Read the model definition and answer for the solid it produces. Units are mm, in the model's axes. Face numbers are marked on the shaded views. A direction names the side the tool comes from. Give positions to 0.01 mm unless a question says otherwise; leave off trailing zeros. Order: outer loops, then holes, each group sorted by start corner. A loop starts at its lowest first (then second) coordinate and runs counter-clockwise, first axis right, second up. Notation, with made-up numbers: (18.25, -28) - (71.25, -28) arc R19 cw to (71.25, -14) - close; hole circle Ø8 at (-4.75, 7.25). An arc over 180 degrees is marked (long way). One line per item, written item: value. Start each with the question number.
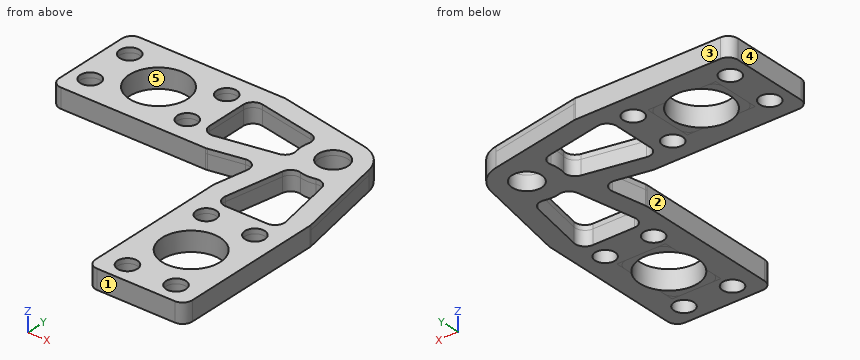
```python
from build123d import *

# Parameters (mm, degrees)
EXTRUDE_1_DEPTH         = 3
SKETCH_2_R              = 2.05
CUT_EXTRUDE_1_DEPTH     = 10
CUT_EXTRUDE_2_DEPTH     = 10
SKETCH_4_R              = 3.05
CUT_EXTRUDE_3_DEPTH     = 10
SKETCH_5_W              = 14
SKETCH_5_H              = 10
SKETCH_5_W_2            = 10
SKETCH_5_H_2            = 14
CUT_EXTRUDE_4_DEPTH     = 10
FILLET_1_R              = 2
FILLET_2_R              = 2
MOVE_START              = 3
MOVE_FACE_1_OUTLINE_R   = 2.05
MOVE_FACE_1_OUTLINE_R_2 = 3.05
MOVE_FACE_1_DEPTH       = 1
SKETCH_9_W              = 14
SKETCH_9_H              = 10
SKETCH_9_W_2            = 10
SKETCH_9_H_2            = 14
EXTRUDE_2_DEPTH         = 4
SKETCH_14_R             = 6
SKETCH_14_R_2           = 2.05
CUT_EXTRUDE_8_DEPTH     = 10


# Read off the part's stored shape, not the designer's step: 移动面1
with BuildPart() as part:
    # 草图1 → 凸台-拉伸1 (new body)
    with BuildSketch(Plane.XY):
        Polygon((-50, 10), (10, 10), (10, -50), (-10, -50), (-10, -10), (-50, -10), align=None)
    extrude(amount=EXTRUDE_1_DEPTH)

    # 草图2 → 切除-拉伸1 (cut)
    with BuildSketch(Plane.XY.offset(3)):
        with Locations((-26, -5)):
            Circle(SKETCH_2_R)
        with Locations((-46, 5)):
            Circle(SKETCH_2_R)
        with Locations((-46, -5)):
            Circle(SKETCH_2_R)
        with Locations((-26, 5)):
            Circle(SKETCH_2_R)
        with Locations((5, -26)):
            Circle(SKETCH_2_R)
        with Locations((-5, -46)):
            Circle(SKETCH_2_R)
        with Locations((5, -46)):
            Circle(SKETCH_2_R)
        with Locations((-5, -26)):
            Circle(SKETCH_2_R)
    extrude(amount=-CUT_EXTRUDE_1_DEPTH, mode=Mode.SUBTRACT)

    # 草图3 → 切除-拉伸2 (cut)
    with BuildSketch(Plane.XY.offset(3)):
        with BuildLine():
            Line((-18, 10), (1.20164514, 6.387961252))
            ThreePointArc((1.20164514, 6.387961252), (4.596194078, 4.596194078), (6.387961252, 1.20164514))
            Line((6.387961252, 1.20164514), (10, -18))
            Line((10, -18), (10, 10))
            Line((10, 10), (-18, 10))
        make_face()
        Polygon((-18, -10), (-8.146437488, -8.146437488), (-10, -18), align=None)
    extrude(amount=-CUT_EXTRUDE_2_DEPTH, mode=Mode.SUBTRACT)

    # 草图4 → 切除-拉伸3 (cut)
    with BuildSketch(Plane.XY.offset(3)):
        Circle(SKETCH_4_R)
    extrude(amount=-CUT_EXTRUDE_3_DEPTH, mode=Mode.SUBTRACT)

    # 草图5 → 切除-拉伸4 (cut)
    with BuildSketch(Plane.XY.offset(3)):
        with Locations((-36, 0)):
            Rectangle(SKETCH_5_W, SKETCH_5_H)
        with BuildLine():
            Line((-22, 6.682287415), (-22, -6.682287415))
            Line((-22, -6.682287415), (-5.43440841, -3.566119072))
            ThreePointArc((-5.43440841, -3.566119072), (-6.5, 0), (-5.43440841, 3.566119072))
            Line((-5.43440841, 3.566119072), (-22, 6.682287415))
        make_face()
        with BuildLine():
            Line((3.566119072, -5.43440841), (6.682287415, -22))
            Line((6.682287415, -22), (-6.682287415, -22))
            Line((-6.682287415, -22), (-3.566119072, -5.43440841))
            ThreePointArc((-3.566119072, -5.43440841), (0, -6.5), (3.566119072, -5.43440841))
        make_face()
        with Locations((0, -36)):
            Rectangle(SKETCH_5_W_2, SKETCH_5_H_2)
    extrude(amount=-CUT_EXTRUDE_4_DEPTH, mode=Mode.SUBTRACT)

    # 圆角1
    fillet_1_edges = [part.edges().sort_by_distance(p)[0] for p in [
        (-29, 5, 1.5),
        (-29, -5, 1.5),
        (-43, -5, 1.5),
        (-43, 5, 1.5),
        (-3.566119072, -5.43440841, 1.5),
        (3.566119072, -5.43440841, 1.5),
        (6.682287415, -22, 1.5),
        (-6.682287415, -22, 1.5),
        (5, -43, 1.5),
        (-5, -43, 1.5),
        (-5, -29, 1.5),
        (5, -29, 1.5),
        (-22, 6.682287415, 1.5),
        (-5.43440841, 3.566119072, 1.5),
        (-5.43440841, -3.566119072, 1.5),
        (-22, -6.682287415, 1.5),
    ]]
    fillet(fillet_1_edges, radius=FILLET_1_R)

    # 圆角2
    fillet_2_edges = [part.edges().sort_by_distance(p)[0] for p in [
        (-50, 10, 1.5),
        (10, -50, 1.5),
        (-10, -50, 1.5),
        (-50, -10, 1.5),
        (-18, -10, 1.5),
        (-8.146437488, -8.146437488, 1.5),
        (-10, -18, 1.5),
        (-18, 10, 1.5),
        (10, -18, 1.5),
    ]]
    fillet(fillet_2_edges, radius=FILLET_2_R)

    # Move Face 1 outline → Move Face 1 (add)
    with BuildSketch(Plane.XY.offset(MOVE_START)):
        with BuildLine():
            Line((-50, 8), (-50, -8))
            ThreePointArc((-50, -8), (-49.414213562, -9.414213562), (-48, -10))
            Line((-48, -10), (-18.186475598, -10))
            ThreePointArc((-18.186475598, -10), (-18.000805296, -9.991362985), (-17.816738632, -9.965526539))
            Line((-17.816738632, -9.965526539), (-11.022770604, -8.687507099))
            ThreePointArc((-11.022770604, -8.687507099), (-9.238820076, -9.238820076), (-8.687507099, -11.022770604))
            Line((-8.687507099, -11.022770604), (-9.965526539, -17.816738632))
            ThreePointArc((-9.965526539, -17.816738632), (-9.991362985, -18.000805296), (-10, -18.186475598))
            Line((-10, -18.186475598), (-10, -48))
            ThreePointArc((-10, -48), (-9.414213562, -49.414213562), (-8, -50))
            Line((-8, -50), (8, -50))
            ThreePointArc((8, -50), (9.414213562, -49.414213562), (10, -48))
            Line((10, -48), (10, -18.186475598))
            ThreePointArc((10, -18.186475598), (9.991362985, -18.000805296), (9.965526539, -17.816738632))
            Line((9.965526539, -17.816738632), (6.387961252, 1.20164514))
            ThreePointArc((6.387961252, 1.20164514), (4.596194078, 4.596194078), (1.20164514, 6.387961252))
            Line((1.20164514, 6.387961252), (-17.816738632, 9.965526539))
            ThreePointArc((-17.816738632, 9.965526539), (-18.000805296, 9.991362985), (-18.186475598, 10))
            Line((-18.186475598, 10), (-48, 10))
            ThreePointArc((-48, 10), (-49.414213562, 9.414213562), (-50, 8))
        make_face()
        with Locations((-5, -46)):
            Circle(MOVE_FACE_1_OUTLINE_R, mode=Mode.SUBTRACT)
        with Locations((5, -46)):
            Circle(MOVE_FACE_1_OUTLINE_R, mode=Mode.SUBTRACT)
        with BuildLine():
            Line((3, -43), (-3, -43))
            ThreePointArc((-3, -43), (-4.414213562, -42.414213562), (-5, -41))
            Line((-5, -41), (-5, -31))
            ThreePointArc((-5, -31), (-4.414213562, -29.585786438), (-3, -29))
            Line((-3, -29), (3, -29))
            ThreePointArc((3, -29), (4.414213562, -29.585786438), (5, -31))
            Line((5, -31), (5, -41))
            ThreePointArc((5, -41), (4.414213562, -42.414213562), (3, -43))
        make_face(mode=Mode.SUBTRACT)
        with Locations((-5, -26)):
            Circle(MOVE_FACE_1_OUTLINE_R, mode=Mode.SUBTRACT)
        with Locations((5, -26)):
            Circle(MOVE_FACE_1_OUTLINE_R, mode=Mode.SUBTRACT)
        with Locations((-46, -5)):
            Circle(MOVE_FACE_1_OUTLINE_R, mode=Mode.SUBTRACT)
        with BuildLine():
            Line((-29, 3), (-29, -3))
            ThreePointArc((-29, -3), (-29.585786438, -4.414213562), (-31, -5))
            Line((-31, -5), (-41, -5))
            ThreePointArc((-41, -5), (-42.414213562, -4.414213562), (-43, -3))
            Line((-43, -3), (-43, 3))
            ThreePointArc((-43, 3), (-42.414213562, 4.414213562), (-41, 5))
            Line((-41, 5), (-31, 5))
            ThreePointArc((-31, 5), (-29.585786438, 4.414213562), (-29, 3))
        make_face(mode=Mode.SUBTRACT)
        with Locations((-46, 5)):
            Circle(MOVE_FACE_1_OUTLINE_R, mode=Mode.SUBTRACT)
        with Locations((-26, -5)):
            Circle(MOVE_FACE_1_OUTLINE_R, mode=Mode.SUBTRACT)
        with Locations((-26, 5)):
            Circle(MOVE_FACE_1_OUTLINE_R, mode=Mode.SUBTRACT)
        with BuildLine():
            ThreePointArc((-4.02556927, -7.876851659), (-3.139359655, -6.562820535), (-1.575326794, -6.306214831))
            ThreePointArc((-1.575326794, -6.306214831), (0, -6.5), (1.575326794, -6.306214831))
            ThreePointArc((1.575326794, -6.306214831), (3.139359655, -6.562820535), (4.02556927, -7.876851659))
            Line((4.02556927, -7.876851659), (6.236514061, -19.630263034))
            ThreePointArc((6.236514061, -19.630263034), (5.810382522, -21.276817541), (4.270987522, -22))
            Line((4.270987522, -22), (-4.270987522, -22))
            ThreePointArc((-4.270987522, -22), (-5.810382522, -21.276817541), (-6.236514061, -19.630263034))
            Line((-6.236514061, -19.630263034), (-4.02556927, -7.876851659))
        make_face(mode=Mode.SUBTRACT)
        with BuildLine():
            ThreePointArc((-7.876851659, 4.02556927), (-6.562820535, 3.139359655), (-6.306214831, 1.575326794))
            ThreePointArc((-6.306214831, 1.575326794), (-6.5, 0), (-6.306214831, -1.575326794))
            ThreePointArc((-6.306214831, -1.575326794), (-6.562820535, -3.139359655), (-7.876851659, -4.02556927))
            Line((-7.876851659, -4.02556927), (-19.630263034, -6.236514061))
            ThreePointArc((-19.630263034, -6.236514061), (-21.276817541, -5.810382522), (-22, -4.270987522))
            Line((-22, -4.270987522), (-22, 4.270987522))
            ThreePointArc((-22, 4.270987522), (-21.276817541, 5.810382522), (-19.630263034, 6.236514061))
            Line((-19.630263034, 6.236514061), (-7.876851659, 4.02556927))
        make_face(mode=Mode.SUBTRACT)
        Circle(MOVE_FACE_1_OUTLINE_R_2, mode=Mode.SUBTRACT)
    extrude(amount=MOVE_FACE_1_DEPTH)

    # 草图9 → 凸台-拉伸2 (add)
    with BuildSketch(Plane.XY.offset(4)):
        with Locations((-36, 0)):
            Rectangle(SKETCH_9_W, SKETCH_9_H)
        with Locations((0, -36)):
            Rectangle(SKETCH_9_W_2, SKETCH_9_H_2)
    extrude(amount=-EXTRUDE_2_DEPTH)

    # 草图14 → 切除-拉伸8 (cut)
    with BuildSketch(Plane.XY.offset(4)):
        with Locations((0, -36)):
            Circle(SKETCH_14_R)
        with Locations((5, -26)):
            Circle(SKETCH_14_R_2)
        with Locations((-5, -26)):
            Circle(SKETCH_14_R_2)
        with Locations((-36, 0)):
            Circle(SKETCH_14_R)
    extrude(amount=-CUT_EXTRUDE_8_DEPTH, mode=Mode.SUBTRACT)


solid = part.part
```
1) Find the intervals of material crossed by probe 1 along Y at (x, z) = (-26, 1.7); probe 2 along Y at (x, z) = (-36, 0.9); probe 3 along X at (y, z) = (0.5, 0.5), in increasing order. Write a range as from..to.
2) For the marked faces 1 and 2, determine the directions among +Z, -Z, +X, -X, +Y, -Y from which every point of the face is accessible in a straight line to the end or side of a thin tool.
3) The mould has two halves that part along X. Classify the marked faces 3, 4 and 5: +X half, -X half, draft (parallel to the pull), parting line (faces both ways), or undercut.
4) Each of these flat-tipped pins is pushed along its axis until it touches: pin 1 (5.5 mm diameter, centred on x = -26, y = 5, fed in from +Z); pin 2 (2 mm diameter, centred on x = -41.5, z = 2.5, fed in from -Y); pin 3 (0.9 mm diameter, centred on y = 0, z = 1.5, fed in from +X); pin 4 (1.1 mm diameter, centred on x = -1, z = 3.5, fed in from +Y). Where does it stop, or does it pass through?
5) Section A-A on x = -36 is taken. Write down the section's boundary in (y, z).
6) Section B-B on y = -46 is taken. Write down the section's boundary in (x, z).
7) Section D-D on z = 0.95 is taken. Give the number of separate pieces and of enclosed holes in the cut face, plus the area to 3 significant figures.
Solved:
1. probe 1: y = -10..-7.05, -2.95..2.95, 7.05..10
1. probe 2: y = -10..-6, 6..10
1. probe 3: x = -50..-41.98, -30.02..-22, -6.48..-3.01, 3.01..6.52
2. face 1: +Z, -Z, +X, -X, -Y
2. face 2: +Z, -Z, -X, -Y
3. face 3: draft
3. face 4: -X half
3. face 5: undercut
4. pin 1: stops at z = 4
4. pin 2: stops at y = -10
4. pin 3: stops at x = 6.7
4. pin 4: stops at y = 6.91
5. outline: (-10, 0) - (-6, 0) - (-6, 4) - (-10, 4) - close; (6, 0) - (10, 0) - (10, 4) - (6, 4) - close
6. outline: (-10, 0) - (-7.05, 0) - (-7.05, 4) - (-10, 4) - close; (-2.95, 0) - (2.95, 0) - (2.95, 4) - (-2.95, 4) - close; (7.05, 0) - (10, 0) - (10, 4) - (7.05, 4) - close
7. separate pieces: 1
7. enclosed holes: 13
7. area: 1,180 mm2
